The listing builds one solid part. Answer for the finished solid, in the listing's coordinates (mm). A direction names the side the tool comes from. Round coordinates to 2 decimals unless told otherwise and drop trailing zeros. Loops run counter-clockwise (first coordinate to the right, second up) from the corner with the lowest first, then second, coordinate; pieces in that order, holes last. Notation, with made-up numbers: (79.5, 61.25) -> (119.5, 61.25) arc R15 cw to (119.5, 71.25) -> close; hole circle Ø11 at (-31, -18.5). An arc over 180 degrees is marked (long way). Use a Markdown table: item, result. Add a question column.
Q1. Which of the six approach directions +Z, -Z, +X, -X, +Y, -Y give full straight-line access (tool end or side, diameter ignored) to faces 1 (the flat face through (9, -9, 0)), 2 (the cylindrical face through (6.37, 0.14, 14.12)), 3 (the flat face through (0, 4, 2))?
Q2. Section A-A on x = 0 is taken. Give the vertices of the cut face in (y, z), then the cut area to 4 significant figures.
Q3. Section D-D on y = -6 is taken. Give the vertices of the cut face in (x, z).
Q4. Consider line 1 (Y direction, x = 0, z = -9.75); line 2 (X direction, y = -3, z = 9); line 3 (Z direction, x = -1, y = -3.75). Determine where each line is inside the solid, lowest interval first.
Q5. Given pin 1 Ø9 at (x, y) = (1, 0.5) entering from +Z; pin 2 Ø1 at (x, y) = (-1, -2.5) entering from +Z, each flat-ended and moving along its own axis, determine where each tip first touches the part or whether it passes through.
Q6. Section C-C on z = -11.25 is taken. Give the vertices of the cut face in (x, y).
Q7. Section B-B on y = 2.25 is taken. Give the vertices of the cut face in (x, z).
Q8. For a pull along Y with two mould halves and no side action, classify faces 4 (the flat face through (-3.48, 1.97, 2.48)), 5 (the flat face through (0, 10, -4)), 6 (the flat face through (10, 0, 0)) as released by +Y, released by -Y, zero draft, split by the parting line, or undercut.
from build123d import *

# Parameters (mm, degrees)
F0_W        = 20
F0_H        = 20
F0_R        = 2.75
F1_DEPTH    = 15
F2_DEPTH    = 15
F4_DEPTH    = 20
F5_T1_DEPTH = 33.2973278516
F6_SIZE     = 2


# Not quite as in the source:
# - a fillet or chamfer that OpenCascade refuses, or shapes differently, is made with other operations: its cross-section is extruded or revolved along the edge and cut away or added


with BuildPart() as f1:
    # F0 (on Top) → F1 (new body)
    with BuildSketch(Plane.XY):
        Rectangle(F0_W, F0_H)
        Polygon((-4.6188021535, 0), (-2.3094010768, 4), (2.3094010768, 4), (4.6188021535, 0), (2.3094010768, -4), (-2.3094010768, -4), align=None, mode=Mode.SUBTRACT)
        Polygon((2.3094010768, 4), (-2.3094010768, 4), (-4.6188021535, 0), (-2.3094010768, -4), (2.3094010768, -4), (4.6188021535, 0), align=None)
        Circle(F0_R, mode=Mode.SUBTRACT)
    extrude(amount=-F1_DEPTH)

    # F0 (on Top) → F2 (join)
    with BuildSketch(Plane.XY):
        Rectangle(F0_W, F0_H)
        Polygon((-4.6188021535, 0), (-2.3094010768, 4), (2.3094010768, 4), (4.6188021535, 0), (2.3094010768, -4), (-2.3094010768, -4), align=None, mode=Mode.SUBTRACT)
    extrude(amount=F2_DEPTH)

    # F3 (on face) → F4 (cut, through all)
    with BuildSketch(Plane.XZ.offset(10)):
        with BuildLine():
            ThreePointArc((-4.5, 11.7041634566), (-1.40312152, 3.9409734138), (5.25, 9))
            ThreePointArc((5.25, 9), (5.0590265862, 10.40312152), (4.5, 11.7041634566))
            ThreePointArc((4.5, 11.7041634566), (0, 14.25), (-4.5, 11.7041634566))
        make_face()
        with BuildLine():
            ThreePointArc((-4.5, 11.7041634566), (0, 14.25), (4.5, 11.7041634566))
            Line((4.5, 11.7041634566), (4.5, 15))
            Line((4.5, 15), (-4.5, 15))
            Line((-4.5, 15), (-4.5, 11.7041634566))
        make_face()
    extrude(amount=-F4_DEPTH, mode=Mode.SUBTRACT)

    # F5: fillet of radius 5 on 2 edges, made by hand

    # F5_s2 → F5_t1 (cut)
    with BuildSketch(Plane.XZ.offset(-11.5457782428)):
        with BuildLine():
            ThreePointArc((-9.2006198435, 15), (-6.330151004, 14.0939478064), (-4.5, 11.7041634566))
            Line((-4.5, 11.7041634566), (-4.5, 15))
            Line((-4.5, 15), (-9.2006198435, 15))
        make_face()
        with BuildLine():
            ThreePointArc((9.2006198435, 15), (6.330151004, 14.0939478064), (4.5, 11.7041634566))
            Line((4.5, 11.7041634566), (4.5, 15))
            Line((4.5, 15), (9.2006198435, 15))
        make_face()
    extrude(amount=F5_T1_DEPTH, mode=Mode.SUBTRACT)

    # F6
    f6_edges = [f1.edges().sort_by_distance(p)[0] for p in [
        (-10, -10, 0),
        (10, -10, 0),
        (-10, 10, 0),
        (10, 10, 0),
    ]]
    chamfer(f6_edges, length=F6_SIZE)


solid = f1.part
Checked values:
| question | item | result |
|---|---|---|
| 1 | face 1 | +Z, -Z, +X, -Y |
| 1 | face 2 | +Z, +Y, -Y |
| 1 | face 3 | +Z |
| 2 | outline | (-10, -15) -> (-2.75, -15) -> (-2.75, 0) -> (-4, 0) -> (-4, 3.75) -> (-10, 3.75) -> close; (2.75, -15) -> (10, -15) -> (10, 3.75) -> (4, 3.75) -> (4, 0) -> (2.75, 0) -> close |
| 2 | area | 262.5 mm2 |
| 3 | outline | (-10, -15) -> (10, -15) -> (10, 15) -> (9.2, 15) arc R5 ccw to (4.5, 11.7) arc R5.25 cw (long way) to (-4.5, 11.7) arc R5 ccw to (-9.2, 15) -> (-10, 15) -> close |
| 4 | line 1 | y = -10 to -2.75, 2.75 to 10 |
| 4 | line 2 | x = -10 to -5.25, 5.25 to 10 |
| 4 | line 3 | z = -15 to 0 |
| 5 | pin 1 | stops at z = 13.36 |
| 5 | pin 2 | stops at z = 0 |
| 6 | outline | (-10, -8) -> (-8, -10) -> (8, -10) -> (10, -8) -> (10, 8) -> (8, 10) -> (-8, 10) -> (-10, 8) -> close; hole circle Ø5.5 at (0, 0) |
| 7 | outline | (-10, -15) -> (-1.58, -15) -> (-1.58, 0) -> (-3.32, 0) -> (-3.32, 4.93) arc R5.25 cw to (-4.5, 11.7) arc R5 ccw to (-9.2, 15) -> (-10, 15) -> close; (1.58, -15) -> (10, -15) -> (10, 15) -> (9.2, 15) arc R5 ccw to (4.5, 11.7) arc R5.25 cw to (3.32, 4.93) -> (3.32, 0) -> (1.58, 0) -> close |
| 8 | face 4 | undercut |
| 8 | face 5 | released by +Y |
| 8 | face 6 | zero draft |
